```python
from build123d import *

# Parameters (mm, degrees)
CYLINDER003_R     = 1.8
CYLINDER003_DEPTH = 40
ARRAY004_Y_COUNT  = 2
ARRAY004_Y_PITCH  = 71
CYLINDER002_R     = 1
CYLINDER002_DEPTH = 100
ARRAY003_X_COUNT  = 2
ARRAY003_X_PITCH  = 43
ARRAY003_Y_COUNT  = 2
ARRAY003_Y_PITCH  = 72
BOX004_W          = 107
BOX004_H          = 80
BOX004_DEPTH      = 3
FILLET001_R       = 2


with BuildPart() as body_corners:
    # Cylinder003 → Cylinder003 (new body)
    with BuildSketch(Plane(origin=(99, -4.5, -15), x_dir=(1, 0, 0), z_dir=(0, 0, 1))):
        Circle(CYLINDER003_R)
    extrude(amount=CYLINDER003_DEPTH)

    # Array004 Y: Body corners ×2


with BuildPart() as body_corners_1:
    add(body_corners.part)
    with Locations(*[(0, i * ARRAY004_Y_PITCH, 0) for i in range(1, ARRAY004_Y_COUNT)]):
        add(body_corners.part)


with BuildPart() as fusion002:
    # Cylinder002 → Cylinder002 (new body)
    with BuildSketch(Plane(origin=(13, -4, -15), x_dir=(1, 0, 0), z_dir=(0, 0, 1))):
        Circle(CYLINDER002_R)
    extrude(amount=CYLINDER002_DEPTH)

    # Array003 X: Fusion002 ×2


with BuildPart() as fusion002_1:
    add(fusion002.part)
    with Locations(*[(i * ARRAY003_X_PITCH, 0, 0) for i in range(1, ARRAY003_X_COUNT)]):
        add(fusion002.part)

    # Array003 Y: Fusion002 ×2


with BuildPart() as fusion002_2:
    add(fusion002_1.part)
    with Locations(*[(0, i * ARRAY003_Y_PITCH, 0) for i in range(1, ARRAY003_Y_COUNT)]):
        add(fusion002_1.part)

    # Fusion002: union Body corners
    add(body_corners_1.part)


with BuildPart() as body006:
    # Box004 → Box004 (new body)
    with BuildSketch(Plane(origin=(-3, -8.5, -3), x_dir=(1, 0, 0), z_dir=(0, 0, 1))):
        with Locations((53.5, 40)):
            Rectangle(BOX004_W, BOX004_H)
    extrude(amount=BOX004_DEPTH)

    # Fillet001
    fillet001_edges = [body006.edges().sort_by_distance(p)[0] for p in [
        (-3, -8.5, -1.5),
        (-3, 71.5, -1.5),
        (104, -8.5, -1.5),
        (104, 71.5, -1.5),
    ]]
    fillet(fillet001_edges, radius=FILLET001_R)

    # Cut002: cut Fusion002
    add(fusion002_2.part, mode=Mode.SUBTRACT)


solid = body006.part
```
The listing builds one solid part. Answer for the finished solid, in the listing's coordinates (mm). Round coordinates to 2 decimals unless told otherwise and drop trailing zeros. Loops run counter-clockwise (first coordinate to the right, second up) from the corner with the lowest first, then second, coordinate; pieces in that order, holes last. Notation, with made-up numbers: (52, 20.5) - (76, 20.5) arc R11 cw to (76, 24.5) - close; hole circle Ø6 at (70.5, 45.25). An arc over 180 degrees is marked (long way). Use one line per item in the form item = value. Start each with the question number.
1. Given pin 1 Ø1.2 at (x, y) = (56, 68) entering from +Z, flat-ended and moving along its own axis, determine where the tip first touches the part or whether it passes through.
2. Consider line 1 (Y direction, x = 99, z = -1.45); line 2 (X direction, y = -4, z = -1); line 3 (X direction, y = 66.5, z = -1.05). Determine where each line is inside the solid, lowest interval first. Write a range as [from, to].
3. For a pull along X with two mould halves and no side action, classify faces 1 (the face through (97.673, 67.717, -1.521)), 2 (the face through (50, -8.5, -2)), 3 (the face through (104, 31, -2)) as pulls with the +X half, pulls with the -X half, needs draft (parallel to the pull), parting line crosses it, or undercut.
4. The part is cut by section A-A on x = 99. Determine the outline of the cut face in (y, z), then the cut area to 3 significant figures.
Geometry check:
q1.pin_1 = through
q2.line_1 = [-8.5, -6.3], [-2.7, 64.7], [68.3, 71.5]
q2.line_2 = [-3, 12], [14, 55], [57, 97.27], [100.73, 104]
q2.line_3 = [-3, 97.2], [100.8, 104]
q3.face_1 = undercut
q3.face_2 = needs draft
q3.face_3 = pulls with the +X half
q4.outline = (-8.5, -3) - (-6.3, -3) - (-6.3, 0) - (-8.5, 0) - close; (-2.7, -3) - (64.7, -3) - (64.7, 0) - (-2.7, 0) - close; (68.3, -3) - (71.5, -3) - (71.5, 0) - (68.3, 0) - close
q4.area = 218 mm^2
